Geometry: final body of the model. Coordinates: model frame, mm. Round coordinates to 2 decimals unless told otherwise and drop trailing zeros. Loops run counter-clockwise (first coordinate to the right, second up) from the corner with the lowest first, then second, coordinate; pieces in that order, holes last. Notation, with made-up numbers: M -34.5,82.25 L 2.5,82.25 A16 cw 2.5,97.25 Z; hole C 16.5,-29 d4. An arc over 180 degrees is marked long. Answer as a JSON object with one key per item and string values.
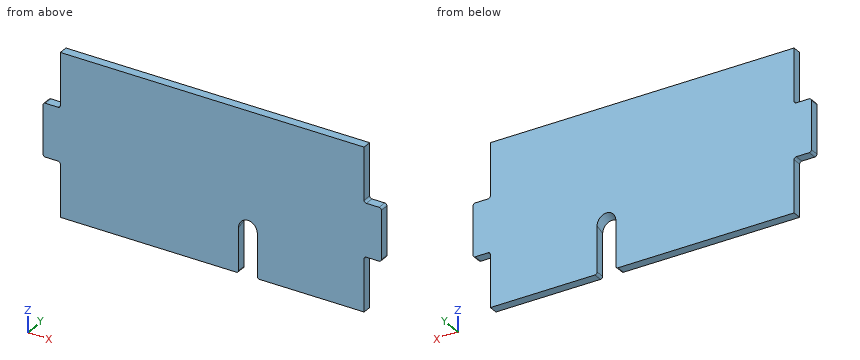
from build123d import *

# Parameters (mm, degrees)
BOSS_EXTRUDE1_DEPTH     = 6.35
CAVITY1_START           = -18.343561252
CAVITY1_OUTLINE_R       = 12.7
CAVITY1_DEPTH           = 21.704189785
CUT_EXTRUDE1_REACH      = 334.451
CUT_EXTRUDE1_END_RADIUS = 12.7
SKETCH4_W               = 25.4
SKETCH4_H               = 12.7
MOVE_FACE_SLOT_BY       = 0.762
MOVE_FACE_SLOT_2_BY     = 0.762
MOVE_FACE_SLOT_3_BY     = 0.762
MOVE_FACE_SLOT_4_BY     = 0.762
MOVE_FACE_SLOT_5_BY     = 0.762
MOVE_FACE_SLOT_6_BY     = 0.762
MOVE_START              = -33.759043645
MOVE_FACE_HOLE_DEPTH    = 37.328109508
FILLET1_R               = 3.175


# Read off the part's stored shape, not the designer's step: Cavity1, Move Face hole
with BuildPart() as part:
    # Sketch1 → Boss-Extrude1 (new, symmetric)
    with BuildSketch(Plane(origin=(0, 0, 0), x_dir=(1, 0, 0), z_dir=(0, 1, 0))):
        Polygon((-215.9, -139.7), (215.9, -139.7), (215.9, -63.5), (241.3, -63.5), (241.3, 12.7), (215.9, 12.7), (215.9, 88.9), (-215.9, 88.9), (-215.9, 12.7), (-241.3, 12.7), (-241.3, -63.5), (-215.9, -63.5), align=None)
    extrude(amount=BOSS_EXTRUDE1_DEPTH, both=True)

    # Cavity1 outline → Cavity1 (cut)
    with BuildSketch(Plane(origin=(0, 0, 0), x_dir=(1, 0, 0), z_dir=(0, 0.9501228611580828, 0.31187585463574896)).offset(CAVITY1_START)):
        with Locations((50.8, 22.822585801)):
            Circle(CAVITY1_OUTLINE_R)
    extrude(amount=CAVITY1_DEPTH, mode=Mode.SUBTRACT)

    # Cut-Extrude1: up to this cylinder (the profile starts outside it)
    cut_extrude1_end = Plane(origin=(50.8, -19.225068271, -30.3312567), z_dir=(0, -0.9501228611580824, -0.3118758546357494)) * Cylinder(CUT_EXTRUDE1_END_RADIUS, 695.302, mode=Mode.PRIVATE)
    # Sketch4 → Cut-Extrude1 (cut, up to the surface)
    with BuildSketch(Plane(origin=(0, 0, -88.9), x_dir=(-1, 0, 0), z_dir=(0, 0, -1)), mode=Mode.PRIVATE) as cut_extrude1_sk1:
        with Locations((-50.8, 0)):
            Rectangle(SKETCH4_W, SKETCH4_H)
    cut_extrude1_tool1 = extrude(cut_extrude1_sk1.sketch, amount=-CUT_EXTRUDE1_REACH, mode=Mode.PRIVATE) - cut_extrude1_end
    add(cut_extrude1_tool1.solids().sort_by_distance((50.8, 0, -88.9))[0], mode=Mode.SUBTRACT)

    # Move Face slot: a face moved inward by 0.762
    extrude(part.faces().sort_by_distance((228.6, 0, 63.5))[0], amount=MOVE_FACE_SLOT_BY, dir=(0, 0, -1), mode=Mode.SUBTRACT)

    # Move Face slot 2: a face moved inward by 0.762
    extrude(part.faces().sort_by_distance((228.6, 0, -12.7))[0], amount=MOVE_FACE_SLOT_2_BY, dir=(0, 0, 1), mode=Mode.SUBTRACT)

    # Move Face slot 3: a face moved inward by 0.762
    extrude(part.faces().sort_by_distance((241.3, 0, 25.4))[0], amount=MOVE_FACE_SLOT_3_BY, dir=(-1, 0, 0), mode=Mode.SUBTRACT)

    # Move Face slot 4: a face moved inward by 0.762
    extrude(part.faces().sort_by_distance((-228.6, 0, 63.5))[0], amount=MOVE_FACE_SLOT_4_BY, dir=(0, 0, -1), mode=Mode.SUBTRACT)

    # Move Face slot 5: a face moved inward by 0.762
    extrude(part.faces().sort_by_distance((-241.3, 0, 25.4))[0], amount=MOVE_FACE_SLOT_5_BY, dir=(1, 0, 0), mode=Mode.SUBTRACT)

    # Move Face slot 6: a face moved inward by 0.762
    extrude(part.faces().sort_by_distance((-228.6, 0, -12.7))[0], amount=MOVE_FACE_SLOT_6_BY, dir=(0, 0, 1), mode=Mode.SUBTRACT)

    # Move Face hole outline → Move Face hole (cut)
    with BuildSketch(Plane(origin=(0, 0, 0), x_dir=(1, 0, 0), z_dir=(0, 0.9501228611580828, 0.31187585463574896)).offset(MOVE_START)):
        with BuildLine():
            ThreePointArc((37.465, 22.822585801), (50.8, 9.487585801), (64.135, 22.822585801))
            Line((64.135, 22.822585801), (64.135, 88))
            Line((64.135, 88), (63.5, 88))
            Line((63.5, 88), (63.5, 22.822585801))
            ThreePointArc((63.5, 22.822585801), (50.8, 10.122585801), (38.1, 22.822585801))
            Line((38.1, 22.822585801), (38.1, 88))
            Line((38.1, 88), (37.465, 88))
            Line((37.465, 88), (37.465, 22.822585801))
        make_face()
    extrude(amount=MOVE_FACE_HOLE_DEPTH, mode=Mode.SUBTRACT)

    # Fillet1
    fillet1_edges = [part.edges().sort_by_distance(p)[0] for p in [
        (-215.9, 0, -11.938),
        (-240.538, 0, -11.938),
        (-240.538, 0, 62.738),
        (-215.9, 0, 62.738),
        (64.135, 0, -88.9),
        (37.465, 0, -88.9),
        (215.9, 0, 62.738),
        (240.538, 0, 62.738),
        (240.538, 0, -11.938),
        (215.9, 0, -11.938),
    ]]
    fillet(fillet1_edges, radius=FILLET1_R)


solid = part.part
1) Section query B-B (z = 71). Return the cut outline in (x, y).
Results:
{"outline": "M -215.9,-6.35 L 215.9,-6.35 L 215.9,6.35 L -215.9,6.35 Z"}
2) Section query A-A (z = -75). Return the cut outline in (x, y) (3 decimals), and give its area (3 significant figures).
Results:
{"outline": "M -215.9,-6.35 L 37.465,-6.35 L 37.465,6.35 L -215.9,6.35 Z; M 64.135,-6.35 L 215.9,-6.35 L 215.9,6.35 L 64.135,6.35 Z", "area": "5,150 mm2"}
3) Ray query, line 1 (X direction, y = 1.5, z = -43.5) (3 decimals); line 2 (X direction, y = 3.5, z = -17.5); line 3 (X direction, y = 1.75, z = 123). Return the intervals inside material, ascending.
Results:
{"line 1": "-215.9 to 37.465, 64.135 to 215.9", "line 2": "-215.9 to 38.48, 63.12 to 215.9", "line 3": "-215.9 to 215.9"}
4) Pin query (flat end, axial travel): P1, Ø6.5, axis at x = 226.5, y = 0.5, coming from the -Z side; P2, Ø6.5, axis at y = -1.5, z = 105, coming from the -X side; P3, Ø6.5, axis at y = 3, z = -61, coming from the +X side. Return the tip coordinate at first contact, or that it passes through.
Results:
{"P1": "z = -11.94", "P2": "x = -215.9", "P3": "x = 215.9"}
